Verification items for the finished model (mm, model axes). Face numbers are marked on the shaded views. A direction names the side the tool comes from. Coordinates: 2 decimals unless noted, no trailing zeros. Order: outer loops, then holes, each group sorted by start corner. A loop starts at its lowest first (then second) coordinate and runs counter-clockwise, first axis right, second up. Notation, with made-up numbers: M 63,75.5 L 115,75.5 A15 ccw 115,99.5 Z; hole C 67.25,77 d6. An arc over 180 degrees is marked long. Return JSON: item names as keys, results as strings.
```python
from build123d import *

# Parameters (mm, degrees)
ESBO_O1_W                = 25
ESBO_O1_H                = 51.5
RESSALTO_EXTRUS_O1_DEPTH = 3
ESBO_O4_W                = 25
ESBO_O4_H                = 3
RESSALTO_EXTRUS_O2_DEPTH = 25
ESBO_O5_R                = 1.65
ESBO_O5_R_2              = 3.7
CORTE_EXTRUS_O1_DEPTH    = 25
ESBO_O7_R                = 1.5
CORTE_EXTRUS_O2_DEPTH    = 25
FILETE1_R                = 5
FILETE2_R                = 2
FILETE3_R                = 1
ESBO_O8_R                = 2.8
CORTE_EXTRUS_O3_DEPTH    = 1.65


with BuildPart() as part:
    # Esboço1 → Ressalto-extrusão1 (new body)
    with BuildSketch(Plane(origin=(0, 0, 0), x_dir=(1, 0, 0), z_dir=(0, 1, 0))):
        with Locations((12.5, 25.75)):
            Rectangle(ESBO_O1_W, ESBO_O1_H)
    extrude(amount=RESSALTO_EXTRUS_O1_DEPTH)

    # Esboço4 → Ressalto-extrusão2 (add)
    with BuildSketch(Plane(origin=(0, 3, 0), x_dir=(1, 0, 0), z_dir=(0, 1, 0))):
        with Locations((12.5, 1.5)):
            Rectangle(ESBO_O4_W, ESBO_O4_H)
    extrude(amount=RESSALTO_EXTRUS_O2_DEPTH)

    # Esboço5 → Corte-extrusão1 (cut)
    with BuildSketch(Plane.XY):
        with Locations((4, 15.5)):
            Circle(ESBO_O5_R)
        with BuildLine():
            ThreePointArc((0, 15.5), (3.661165235, 24.338834765), (12.5, 28))
            Line((12.5, 28), (0, 28))
            Line((0, 28), (0, 15.5))
        make_face()
        with Locations((12.5, 24)):
            Circle(ESBO_O5_R)
        with Locations((12.5, 15.5)):
            Circle(ESBO_O5_R_2)
        with Locations((21, 15.5)):
            Circle(ESBO_O5_R)
        with Locations((12.5, 7)):
            Circle(ESBO_O5_R)
        with BuildLine():
            ThreePointArc((12.5, 28), (21.338834765, 24.338834765), (25, 15.5))
            Line((25, 15.5), (25, 28))
            Line((25, 28), (12.5, 28))
        make_face()
    extrude(amount=-CORTE_EXTRUS_O1_DEPTH, mode=Mode.SUBTRACT)

    # Esboço7 → Corte-extrusão2 (cut)
    with BuildSketch(Plane(origin=(0, 3, 0), x_dir=(1, 0, 0), z_dir=(0, 1, 0))):
        with Locations(Location((12.5, 34.33, 0), (0, 0, 270))):
            Circle(ESBO_O7_R)
        with Locations(Location((12.5, 21.63, 0), (0, 0, 270))):
            Circle(ESBO_O7_R)
        with Locations(Location((12.5, 8.93, 0), (0, 0, 270))):
            Circle(ESBO_O7_R)
        with Locations(Location((12.5, 47.08, 0), (0, 0, 270))):
            Circle(ESBO_O7_R)
    extrude(amount=-CORTE_EXTRUS_O2_DEPTH, mode=Mode.SUBTRACT)

    # Filete1
    filete1_edges = [part.edges().sort_by_distance(p)[0] for p in [
        (0, 1.5, -51.5),
        (25, 1.5, -51.5),
    ]]
    fillet(filete1_edges, radius=FILETE1_R)

    # Filete2
    filete2_edges = [part.edges().sort_by_distance(p)[0] for p in [
        (12.5, 0, 0),
    ]]
    fillet(filete2_edges, radius=FILETE2_R)

    # Filete3
    filete3_edges = [part.edges().sort_by_distance(p)[0] for p in [
        (12.5, 3, -3),
    ]]
    fillet(filete3_edges, radius=FILETE3_R)

    # Esboço8 → Corte-extrusão3 (cut)
    with BuildSketch(Plane(origin=(0, 3, 0), x_dir=(1, 0, 0), z_dir=(0, 1, 0))):
        with Locations(Location((12.5, 47.08, 0), (0, 0, 270))):
            Circle(ESBO_O8_R)
        with Locations(Location((12.5, 34.33, 0), (0, 0, 270))):
            Circle(ESBO_O8_R)
        with Locations(Location((12.5, 21.63, 0), (0, 0, 270))):
            Circle(ESBO_O8_R)
        with Locations(Location((12.5, 8.93, 0), (0, 0, 270))):
            Circle(ESBO_O8_R)
    extrude(amount=-CORTE_EXTRUS_O3_DEPTH, mode=Mode.SUBTRACT)


solid = part.part
```
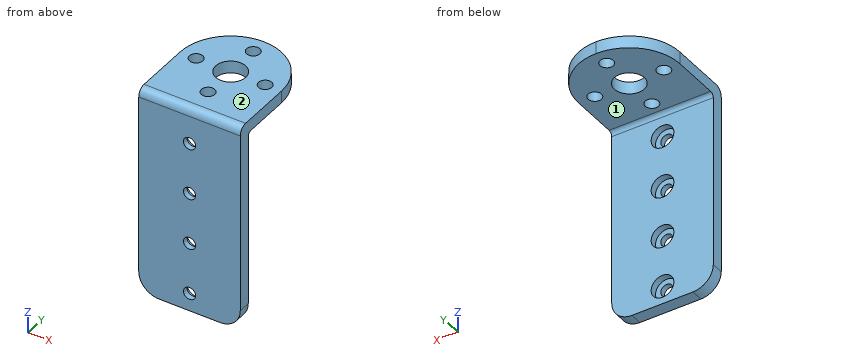
Q1. Cross-section at A-A, the plane z = -8.93. Record the boundary of the cut face in (x, y), and give its area (3 significant figures).
Values:
{"outline": "M 0,0 L 11,0 L 11,1.35 L 9.7,1.35 L 9.7,3 L 0,3 Z; M 14,0 L 25,0 L 25,3 L 15.3,3 L 15.3,1.35 L 14,1.35 Z", "area": "61.7 mm^2"}
Q2. Cross-section at D-D, the plane x = 7. Record the boundary of the cut face in (y, z), and give its area (3 significant figures).
Values:
{"outline": "M 0,-51.5 L 3,-51.5 L 3,-4 A1 cw 4,-3 L 26.72,-3 L 26.72,0 L 2,0 A2 ccw 0,-2 Z", "area": "225 mm^2"}
Q3. Material ranges on line 1 along X through (y, z) = (1.95, -8.93); line 2 along X through (y, z) = (0.5, -34.33); line 3 along Y through (x, z) = (16.25, -43), recorded low to high.
Values:
{"line 1": "0 to 9.7, 15.3 to 25", "line 2": "0 to 11, 14 to 25", "line 3": "0 to 3"}
Q4. Go/stop test with flat-tipped pins: pin 1 (1.5 mm diameter, centred on x = 12.5, z = -38.5, fed in from -Y); pin 2 (2 mm diameter, centred on x = 12.5, y = 14.5, fed in from +Z); pin 3 (4 mm diameter, centred on x = 21, y = 15.5, fed in from -Z); pin 4 (6 mm diameter, centred on x = 11.5, z = -34.5, fed in from +Y). Record where each tip stops, or that it passes through.
Values:
{"pin 1": "y = 0", "pin 2": "through", "pin 3": "z = -3", "pin 4": "y = 3"}
Q5. Cross-section at B-B, the plane y = 7. Record the boundary of the cut face in (x, z).
Values:
{"outline": "M 0,-3 L 10.85,-3 L 10.85,0 L 0,0 Z; M 14.15,-3 L 25,-3 L 25,0 L 14.15,0 Z"}
Q6. Tool access check on the marked faces 1 and 2. Record the directions out of +Z, -Z, +X, -X, +Y, -Y that give a thin tool (end or side, any length) a straight path to the whole face; none if there is none.
Values:
{"face 1": "-Z, +X, -X, +Y", "face 2": "+Z, +X, -X, +Y, -Y"}
Q7. Cross-section at C-C, the plane x = 4. Record the boundary of the cut face in (y, z), and give its area (3 significant figures).
Values:
{"outline": "M 0,-51.4 L 3,-51.4 L 3,-4 A1 cw 4,-3 L 13.85,-3 L 13.85,0 L 2,0 A2 ccw 0,-2 Z; M 17.15,-3 L 24.67,-3 L 24.67,0 L 17.15,0 Z", "area": "209 mm^2"}
